Read the model definition and answer for the solid it produces. Units are mm, in the model's axes. A direction names the side the tool comes from. Round coordinates to 2 decimals unless told otherwise and drop trailing zeros. Order: outer loops, then holes, each group sorted by start corner. A loop starts at its lowest first (then second) coordinate and runs counter-clockwise, first axis right, second up. Notation, with made-up numbers: (1, 75) -> (10, 75) arc R18 cw to (10, 86) -> close; hole circle Ø9 at (-12, 79). An arc over 180 degrees is marked (long way). Use a Markdown table: item, result. Add a question column.
1. Consider L1, parallel to Z at x = 2.75, y = 7.5; L2, parallel to Y at x = 6, z = 3.9; L3, parallel to X at y = 7.5, z = 1. Determine where each line is inside the solid, lowest interval first. Write a range as [from, to].
2. Section D-D, the plane y = 6.5 is taken. Give the vertices of the cut face in (x, z), then the cut area to 3 significant figures.
3. For faces 4 (the face through (5, 5, 0)), 5 (the face through (4.6, 5.6, 3.5)), 6 (the face through (12, 3, 4)), 7 (the face through (5, 5, 5)), determine the directions among +Z, -Z, +X, -X, +Y, -Y from which every point of the face is accessible in a straight line to the end or side of a thin tool.
4. Given pin 1 (1.5 mm diameter, centred on x = 1.5, y = 7, fed in from +Z); pin 2 (1.5 mm diameter, centred on x = 10.5, z = 1.5, fed in from +Y); pin 3 (2.5 mm diameter, centred on x = 6.5, y = 5.5, fed in from -Z), each flat-ended and moving along its own axis, determine where each tip first touches the part or whether it passes through.
5. The mould has two halves that part along Z. Classify faces 1 (the face through (6.1, 0.9, -0.6)), 2 (the face through (0.86, 10.3, 4.24)), 3 (the face through (6.084, 1.485, 1.801)): +Z half, -Z half, draft (parallel to the pull), parting line (faces both ways), or undercut.
6. Section B-B, the plane z = 4.75 is taken. Give the vertices of the cut face in (x, y).
7. Section C-C, the plane x = 6 is taken. Give the number of separate pieces and of enclosed holes in the cut face, then the cut area to 3 significant figures.
8. Section A-A, the plane y = 4.25 is taken. Give the vertices of the cut face in (x, z), then the cut area to 3 significant figures.
```python
from build123d import *

# Parameters (mm, degrees)
SKETCH1_W           = 12
SKETCH1_H           = 5
BOSS_EXTRUDE1_DEPTH = 1.2
SKETCH2_W           = 12
SKETCH2_H           = 1.5
BOSS_EXTRUDE2_DEPTH = 10
FILLET1_R           = 3
FILLET2_R           = 1
SKETCH3_R           = 1.5
CUT_EXTRUDE1_DEPTH  = 18.159254063
BOSS_EXTRUDE3_DEPTH = 12


with BuildPart() as part:
    # Sketch1 → Boss-Extrude1 (new body)
    with BuildSketch(Plane(origin=(0, 0, 0), x_dir=(1, 0, 0), z_dir=(0, 1, 0))):
        with Locations((6, -2.5)):
            Rectangle(SKETCH1_W, SKETCH1_H)
    extrude(amount=BOSS_EXTRUDE1_DEPTH)

    # Sketch2 → Boss-Extrude2 (add)
    with BuildSketch(Plane(origin=(0, 1.2, 0), x_dir=(1, 0, 0), z_dir=(0, 1, 0))):
        with Locations((6, -4.25)):
            Rectangle(SKETCH2_W, SKETCH2_H)
        with Locations((6, -0.75)):
            Rectangle(SKETCH2_W, SKETCH2_H)
    extrude(amount=BOSS_EXTRUDE2_DEPTH)

    # Fillet1
    fillet1_edges = [part.edges().sort_by_distance(p)[0] for p in [
        (0, 11.2, 4.25),
        (12, 11.2, 4.25),
        (12, 11.2, 0.75),
        (0, 11.2, 0.75),
    ]]
    fillet(fillet1_edges, radius=FILLET1_R)

    # Fillet2
    fillet2_edges = [part.edges().sort_by_distance(p)[0] for p in [
        (6, 1.2, 3.5),
        (6, 1.2, 1.5),
    ]]
    fillet(fillet2_edges, radius=FILLET2_R - 0.0001)  # a hair under: the kernel refuses the full size

    # Sketch3 → Cut-Extrude1 (cut, through all)
    with BuildSketch(Plane(origin=(0, 0, 0), x_dir=(-1, 0, 0), z_dir=(0, 0, -1))):
        with Locations((-6, 6.5)):
            Circle(SKETCH3_R)
    extrude(amount=-CUT_EXTRUDE1_DEPTH, mode=Mode.SUBTRACT)

    # Sketch4 → Boss-Extrude3 (add)
    with BuildSketch(Plane(origin=(12, 0, 0), x_dir=(0, 0, -1), z_dir=(1, 0, 0))):
        Polygon((0, 1.5), (1.303058947, 0.196941053), (1.303058947, 0), (0, 0), align=None)
        Polygon((-6.303058947, 0), (-6.303058947, 0.196941053), (-5, 1.5), (-5, 0), align=None)
    extrude(amount=-BOSS_EXTRUDE3_DEPTH)


solid = part.part
```
Verdict:
| question | item | result |
|---|---|---|
| 1 | L1 | z = [0, 1.5], [3.5, 5] |
| 1 | L2 | y = [0, 5], [8, 11.2] |
| 1 | L3 | x = [0, 4.88], [7.12, 12] |
| 2 | outline | (0, 0) -> (4.5, 0) -> (4.5, 1.5) -> (0, 1.5) -> close; (0, 3.5) -> (4.5, 3.5) -> (4.5, 5) -> (0, 5) -> close; (7.5, 0) -> (12, 0) -> (12, 1.5) -> (7.5, 1.5) -> close; (7.5, 3.5) -> (12, 3.5) -> (12, 5) -> (7.5, 5) -> close |
| 2 | area | 27.0 mm2 |
| 3 | face 4 | -Z, +X, -X, +Y |
| 3 | face 5 | +X, -X, +Y |
| 3 | face 6 | +Z, -Z, +X, +Y, -Y |
| 3 | face 7 | +Z, +X, -X, +Y |
| 4 | pin 1 | stops at z = 5 |
| 4 | pin 2 | stops at y = 11.1 |
| 4 | pin 3 | stops at z = 0 |
| 5 | face 1 | -Z half |
| 5 | face 2 | draft |
| 5 | face 3 | undercut |
| 6 | outline | (0, 0) -> (12, 0) -> (12, 8.2) arc R3 ccw to (9, 11.2) -> (3, 11.2) arc R3 ccw to (0, 8.2) -> close; hole circle Ø3 at (6, 6.5) |
| 7 | separate pieces | 3 |
| 7 | enclosed holes | 0 |
| 7 | area | 29.6 mm2 |
| 8 | outline | (0, 0) -> (12, 0) -> (12, 1.5) -> (0, 1.5) -> close; (0, 3.5) -> (12, 3.5) -> (12, 5) -> (0, 5) -> close |
| 8 | area | 36.0 mm2 |
